The listing builds one solid part. Answer for the finished solid, in the listing's coordinates (mm). Round coordinates to 2 decimals unless told otherwise and drop trailing zeros. One line per question, with ' | ' between items.
Autodesk Inventor part; units mm, degrees
ref_plane "side_4d_XY" through (-20, 0, -313.5) normal (-1, 0, 0) x (0, 1, 0)
ref_plane "side_4d_YZ" through (-20, 0, -313.5) normal (0, 1, 0) x (0, 0, -1)
ref_plane "side_4d_ZX" through (-20, 0, -313.5) normal (0, 0, -1) x (-1, 0, 0)
sketch "Skizze_1" plane through (0, 0, 0) normal (0, 0, 1) x (1, 0, 0)
  arc A0 (-20, -17) -> (-17, -20) centre (-17, -17) ccw
  line L0 (-17, -20) -> (-4.1, -20)
  line L1 (-4.1, -20) -> (-4.1, -17)
  line L2 (-4.1, -17) -> (-10.5, -17)
  line L3 (-10.5, -17) -> (-10.5, -13.6627)
  arc A1 (-10.0314, -12.5314) -> (-10.5, -13.6627) centre (-8.9002, -13.6627) ccw
  line L4 (-10.0314, -12.5314) -> (-7.4645, -9.9645)
  arc A2 (-3.9289, -8.5) -> (-7.4645, -9.9645) centre (-3.9289, -13.5) ccw
  line L5 (-3.9289, -8.5) -> (3.9289, -8.5)
  arc A3 (7.4645, -9.9645) -> (3.9289, -8.5) centre (3.9289, -13.5) ccw
  line L6 (7.4645, -9.9645) -> (10.0314, -12.5314)
  arc A4 (10.5, -13.6627) -> (10.0314, -12.5314) centre (8.9002, -13.6627) ccw
  line L7 (10.5, -13.6627) -> (10.5, -17)
  line L8 (10.5, -17) -> (4.1, -17)
  line L9 (4.1, -17) -> (4.1, -20)
  line L10 (4.1, -20) -> (17, -20)
  arc A5 (17, -20) -> (20, -17) centre (17, -17) ccw
  line L11 (20, -17) -> (20, -4.1)
  line L12 (20, -4.1) -> (17, -4.1)
  line L13 (17, -4.1) -> (17, -10.5)
  line L14 (17, -10.5) -> (13.6627, -10.5)
  arc A6 (12.5314, -10.0314) -> (13.6627, -10.5) centre (13.6627, -8.9002) ccw
  line L15 (12.5314, -10.0314) -> (9.9645, -7.4645)
  arc A7 (8.5, -3.9289) -> (9.9645, -7.4645) centre (13.5, -3.9289) ccw
  line L16 (8.5, -3.9289) -> (8.5, 3.9289)
  arc A8 (9.9645, 7.4645) -> (8.5, 3.9289) centre (13.5, 3.9289) ccw
  line L17 (9.9645, 7.4645) -> (12.5314, 10.0314)
  arc A9 (13.6627, 10.5) -> (12.5314, 10.0314) centre (13.6627, 8.9002) ccw
  line L18 (13.6627, 10.5) -> (17, 10.5)
  line L19 (17, 10.5) -> (17, 4.1)
  line L20 (17, 4.1) -> (20, 4.1)
  line L21 (20, 4.1) -> (20, 17)
  arc A10 (20, 17) -> (17, 20) centre (17, 17) ccw
  line L22 (17, 20) -> (4.1, 20)
  line L23 (4.1, 20) -> (4.1, 17)
  line L24 (4.1, 17) -> (10.5, 17)
  line L25 (10.5, 17) -> (10.5, 13.6627)
  arc A11 (10.0314, 12.5314) -> (10.5, 13.6627) centre (8.9002, 13.6627) ccw
  line L26 (10.0314, 12.5314) -> (7.4645, 9.9645)
  arc A12 (3.9289, 8.5) -> (7.4645, 9.9645) centre (3.9289, 13.5) ccw
  line L27 (3.9289, 8.5) -> (-3.9289, 8.5)
  arc A13 (-7.4645, 9.9645) -> (-3.9289, 8.5) centre (-3.9289, 13.5) ccw
  line L28 (-7.4645, 9.9645) -> (-10.0314, 12.5314)
  arc A14 (-10.5, 13.6627) -> (-10.0314, 12.5314) centre (-8.9002, 13.6627) ccw
  line L29 (-10.5, 13.6627) -> (-10.5, 17)
  line L30 (-10.5, 17) -> (-4.1, 17)
  line L31 (-4.1, 17) -> (-4.1, 20)
  line L32 (-4.1, 20) -> (-17, 20)
  arc A15 (-17, 20) -> (-20, 17) centre (-17, 17) ccw
  line L33 (-20, 17) -> (-20, 4.1)
  line L34 (-20, 4.1) -> (-17, 4.1)
  line L35 (-17, 4.1) -> (-17, 10.5)
  line L36 (-17, 10.5) -> (-13.6627, 10.5)
  arc A16 (-12.5314, 10.0314) -> (-13.6627, 10.5) centre (-13.6627, 8.9002) ccw
  line L37 (-12.5314, 10.0314) -> (-9.9645, 7.4645)
  arc A17 (-8.5, 3.9289) -> (-9.9645, 7.4645) centre (-13.5, 3.9289) ccw
  line L38 (-8.5, 3.9289) -> (-8.5, -3.9289)
  arc A18 (-9.9645, -7.4645) -> (-8.5, -3.9289) centre (-13.5, -3.9289) ccw
  line L39 (-9.9645, -7.4645) -> (-12.5314, -10.0314)
  arc A19 (-13.6627, -10.5) -> (-12.5314, -10.0314) centre (-13.6627, -8.9002) ccw
  line L40 (-13.6627, -10.5) -> (-17, -10.5)
  line L41 (-17, -10.5) -> (-17, -4.1)
  line L42 (-17, -4.1) -> (-20, -4.1)
  line L43 (-20, -4.1) -> (-20, -17)
  circle A20 centre (0, 0) radius 6
extrude "Extrusion1" add sketch "Skizze_1" against normal blind 627
sketch "Sketch2" plane through (0, 0, 0) normal (0, 0, 1) x (1, 0, 0)
  point P0 (-15, -15)
hole "Drilling 1" at (-15, -15, 0) direction (0, 0, -1) diameter 5 depth 6000
sketch "Sketch3" plane through (0, 0, 0) normal (0, 0, 1) x (1, 0, 0)
  point P0 (15, -15)
hole "Drilling 2" at (15, -15, 0) direction (0, 0, -1) diameter 5 depth 6000
sketch "Sketch4" plane through (0, 0, 0) normal (0, 0, 1) x (1, 0, 0)
  point P0 (15, 15)
hole "Drilling 3" at (15, 15, 0) direction (0, 0, -1) diameter 5 depth 6000
sketch "Sketch5" plane through (0, 0, 0) normal (0, 0, 1) x (1, 0, 0)
  point P0 (-15, 15)
hole "Drilling 4" at (-15, 15, 0) direction (0, 0, -1) diameter 5 depth 6000
ref_plane "side_4d_XY" through (-20, 0, -313.5) normal (-1, 0, 0) x (0, 1, 0)
ref_plane "side_4d_YZ" through (-20, 0, -313.5) normal (0, 1, 0) x (0, 0, -1)
ref_plane "side_4d_ZX" through (-20, 0, -313.5) normal (0, 0, -1) x (-1, 0, 0)
ref_plane "side_1a_XY" through (0, 20, -313.5) normal (0, 1, 0) x (1, 0, 0)
ref_plane "side_1a_YZ" through (0, 20, -313.5) normal (1, 0, 0) x (0, 0, -1)
ref_plane "side_1a_ZX" through (0, 20, -313.5) normal (0, 0, -1) x (0, 1, 0)
ref_plane "side_2b_XY" through (20, 0, -313.5) normal (1, 0, 0) x (0, -1, 0)
ref_plane "side_2b_YZ" through (20, 0, -313.5) normal (0, -1, 0) x (0, 0, -1)
ref_plane "side_2b_ZX" through (20, 0, -313.5) normal (0, 0, -1) x (1, 0, 0)
ref_plane "side_3c_XY" through (0, -20, -313.5) normal (0, -1, 0) x (-1, 0, 0)
ref_plane "side_3c_YZ" through (0, -20, -313.5) normal (-1, 0, 0) x (0, 0, -1)
ref_plane "side_3c_ZX" through (0, -20, -313.5) normal (0, 0, -1) x (0, -1, 0)
ref_plane "end_XY" through (0, 0, -627) normal (0, 0, -1) x (1, 0, 0)
ref_plane "end_YZ" through (0, 0, -627) normal (1, 0, 0) x (0, -1, 0)
ref_plane "end_ZX" through (0, 0, -627) normal (0, -1, 0) x (0, 0, -1)
ref_plane "start_XY" through (0, 0, 0) normal (0, 0, 1) x (1, 0, 0)
ref_plane "start_YZ" through (0, 0, 0) normal (1, 0, 0) x (0, 1, 0)
ref_plane "start_ZX" through (0, 0, 0) normal (0, 1, 0) x (0, 0, 1)
properties part number "MayTec 1.11.040040.43S_Profile 40x40, 4E, S_627_Detail_(0;0,0,0)"
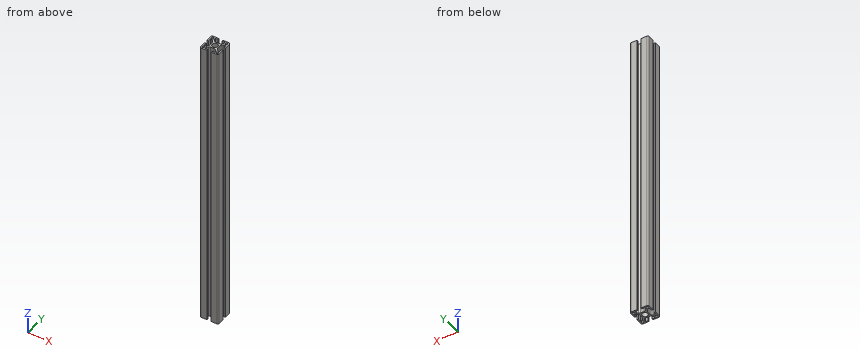
Q1. A cutting plane is placed at A-A on z = -359. Give the number of separate pieces and of enclosed holes in the cut face, plus the area to 3 significant figures.
Numbers:
separate pieces: 1 | enclosed holes: 5 | area: 674 mm^2
Q2. Find the intervals of material crossed by line 1 (Y direction, x = 15, z = -165); line 2 (Y direction, x = 10, z = -436.5), in increasing order. Write a range as from..to.
Numbers:
line 1: -20..-17.5, -12.5..-10.5, 10.5..12.5, 17.5..20 | line 2: -20..-17, -12.5..-7.5, 7.5..12.5, 17..20
Q3. Given pin 1 Ø0.9 at (x, z) = (-18, -211) entering from -Y; pin 2 Ø0.9 at (x, z) = (-18, -377) entering from +Y; pin 3 Ø4 at (y, z) = (-0.5, -559) entering from -X, each flat-ended and moving along its own axis, determine where each tip first touches the part or whether it passes through.
Numbers:
pin 1: y = -19.95 | pin 2: y = 19.95 | pin 3: x = -8.5
